Work out the finished part from the listing and answer in its coordinate system (mm). A direction names the side the tool comes from. Coordinates: 2 decimals unless noted, no trailing zeros. Order: outer loops, then holes, each group sorted by start corner. A loop starts at its lowest first (then second) coordinate and runs counter-clockwise, first axis right, second up. Notation, with made-up numbers: M 46.5,4 L 55.5,4 A11 cw 55.5,10 Z; hole C -39,3 d2. An arc over 180 degrees is marked long. Use a Markdown table: item, result. Add a question column.
from build123d import *

# Parameters (mm, degrees)
F1_DEPTH = 10
F2_DEPTH = 5
F3_D     = 2
F3_DEPTH = 4
F3_TIP   = 0.600860619
F4_R     = 5
F6_D     = 6
F6_DEPTH = 2
F6_TIP   = 1.8025818571
F8_D     = 6
F8_DEPTH = 2
F8_TIP   = 1.8025818571


# Not quite as in the source:
# - a feature names something its author has since deleted; it is built from what else it names


with BuildPart() as f1:
    # F0 (on Top) → F1 (new body)
    with BuildSketch(Plane.XY):
        Polygon((70, 70), (-70, 70), (-70, 15.5), (-68, 15.5), (-68, 68), (68, 68), (68, 15.5), (70, 15.5), align=None)
        Polygon((-68, 68), (-68, 15.5), (-68, 0), (-68, -15.5), (-68, -68), (68, -68), (68, -15.5), (68, 0), (68, 15.5), (68, 68), align=None)
        Polygon((53, -18), (53, -53), (-53, -53), (-53, -18), (-53, 18), (-53, 53), (53, 53), (53, 18), (53, 0), align=None, mode=Mode.SUBTRACT)
        Polygon((-68, 15.5), (-70, 15.5), (-70, -15.5), (-68, -15.5), (-68, 0), align=None)
        Polygon((-68, -15.5), (-70, -15.5), (-70, -70), (70, -70), (70, -15.5), (68, -15.5), (68, -68), (-68, -68), align=None)
        Polygon((70, -15.5), (70, 15.5), (68, 15.5), (68, 0), (68, -15.5), align=None)
        Polygon((-53, 53), (-53, 18), (-51, 18), (-51, 51), (51, 51), (51, 18), (53, 18), (53, 53), align=None)
        Polygon((-53, 18), (-53, -18), (-51, -18), (-51, 0), (-51, 18), align=None)
        Polygon((51, -18), (53, -18), (53, 0), (53, 18), (51, 18), align=None)
        Polygon((-53, -53), (53, -53), (53, -18), (51, -18), (51, -51), (-51, -51), (-51, -18), (-53, -18), align=None)
    extrude(amount=F1_DEPTH)

    # F0 (on Top) → F2 (join)
    with BuildSketch(Plane.XY):
        Polygon((70, 70), (-70, 70), (-70, 15.5), (-68, 15.5), (-68, 68), (68, 68), (68, 15.5), (70, 15.5), align=None)
        Polygon((-68, -15.5), (-70, -15.5), (-70, -70), (70, -70), (70, -15.5), (68, -15.5), (68, -68), (-68, -68), align=None)
        Polygon((-53, -53), (53, -53), (53, -18), (51, -18), (51, -51), (-51, -51), (-51, -18), (-53, -18), align=None)
        Polygon((-53, 53), (-53, 18), (-51, 18), (-51, 51), (51, 51), (51, 18), (53, 18), (53, 53), align=None)
    extrude(amount=-F2_DEPTH)

    # F3
    with Locations(Plane(origin=(0, 0, 0), x_dir=(1, 0, 0), z_dir=(0, 0, -1))):
        with Locations((0, 60.5), (60.5, 0), (0, -60.5), (-60.5, 0), (-60.5, 40), (-40, 60.5), (40, 60.5), (60.5, 40), (60.5, -40), (40, -60.5), (-40, -60.5), (-60.5, -40)):
            Hole(F3_D / 2, depth=F3_DEPTH)
            with Locations((0, 0, -(F3_DEPTH + F3_TIP / 2))):  # 118° drill point
                Cone(0, F3_D / 2, F3_TIP, mode=Mode.SUBTRACT)

    # F4
    f4_edges = [f1.edges().sort_by_distance(p)[0] for p in [
        (-68, -68, -2.5),
        (-53, -53, -2.5),
        (-53, 53, -2.5),
        (53, 53, -2.5),
        (53, -53, -2.5),
        (68, 68, -2.5),
        (-68, 68, -2.5),
        (68, -68, -2.5),
    ]]
    fillet(f4_edges, radius=F4_R)

    # F6 (one way)
    with BuildSketch(Plane.XZ.offset(-51)):
        with Locations((0, 6.5)):
            Circle(F6_D / 2)
    extrude(amount=-F6_DEPTH, mode=Mode.SUBTRACT)
    with Locations(Plane.XZ.offset(-51)):
        with Locations((0, 6.5)):
            with Locations((0, 0, -(F6_DEPTH + F6_TIP / 2))):  # 118° drill point
                Cone(0, F6_D / 2, F6_TIP, mode=Mode.SUBTRACT)

    # F8 (one way)
    with BuildSketch(Plane(origin=(0, -51, 0), x_dir=(-1, 0, 0), z_dir=(0, 1, 0))):
        with Locations((0, 6.5)):
            Circle(F8_D / 2)
    extrude(amount=-F8_DEPTH, mode=Mode.SUBTRACT)
    with Locations(Plane(origin=(0, -51, 0), x_dir=(-1, 0, 0), z_dir=(0, 1, 0))):
        with Locations((0, 6.5)):
            with Locations((0, 0, -(F8_DEPTH + F8_TIP / 2))):  # 118° drill point
                Cone(0, F8_D / 2, F8_TIP, mode=Mode.SUBTRACT)


solid = f1.part
(1) Straight lines are drawn through the part: line 1 (Y direction, x = -40, z = 2.9); line 2 (Y direction, x = -44, z = -2.75). For each, find the intervals that lie inside material, in ascending order.
(2) Given P1, Ø1.8, axis at x = 40, y = -60.5, coming from the -Z side; P2, Ø3, axis at x = 60.5, y = 40, coming from the -Z side, each flat-ended and moving along its own axis, determine where each tip first touches the part or whether it passes through.
(3) A cutting plane is placed at A-A on y = 34. Write down the section's boundary in (x, z), plus the area to 3 significant figures.
(4) The mould has two halves that part along Z. Classify faces 6 (the flat face through (68, -39, -2)), 7 (the flat face through (-28, -52, -5)), 8 (the cylindrical face through (0.65, -51.99, 3.57)): pulls with the +Z half, pulls with the -Z half, needs draft (parallel to the pull), parting line crosses it, or undercut.
(5) Which of the six approach directions +Z, -Z, +X, -X, +Y, -Y give full straight-line access (tool end or side, diameter ignored) to faces 1 (the flat face through (70, -1, 3)), 2 (the cylindrical face through (-66, -67, -3)), 3 (the flat face through (1, 70, 3)), 4 (the flat face through (51, 1, 2)), 5 (the cylindrical face through (-0.65, 51.99, 3.57))?
From the geometry:
| question | item | result |
|---|---|---|
| 1 | line 1 | y = -70 to -61.5, -59.5 to -51, 51 to 59.5, 61.5 to 70 |
| 1 | line 2 | y = -70 to -68, -53 to -51, 51 to 53, 68 to 70 |
| 2 | P1 | stops at z = 4.06 |
| 2 | P2 | stops at z = 0 |
| 3 | outline | M -70,-5 L -68,-5 L -68,0 L -53,0 L -53,-5 L -51,-5 L -51,10 L -70,10 Z; M 51,-5 L 53,-5 L 53,0 L 68,0 L 68,-5 L 70,-5 L 70,10 L 51,10 Z |
| 3 | area | 420 mm2 |
| 4 | face 6 | needs draft |
| 4 | face 7 | pulls with the -Z half |
| 4 | face 8 | undercut |
| 5 | face 1 | +Z, -Z, +X, +Y, -Y |
| 5 | face 2 | -Z |
| 5 | face 3 | +Z, -Z, +X, -X, +Y |
| 5 | face 4 | +Z, -Z |
| 5 | face 5 | none |
